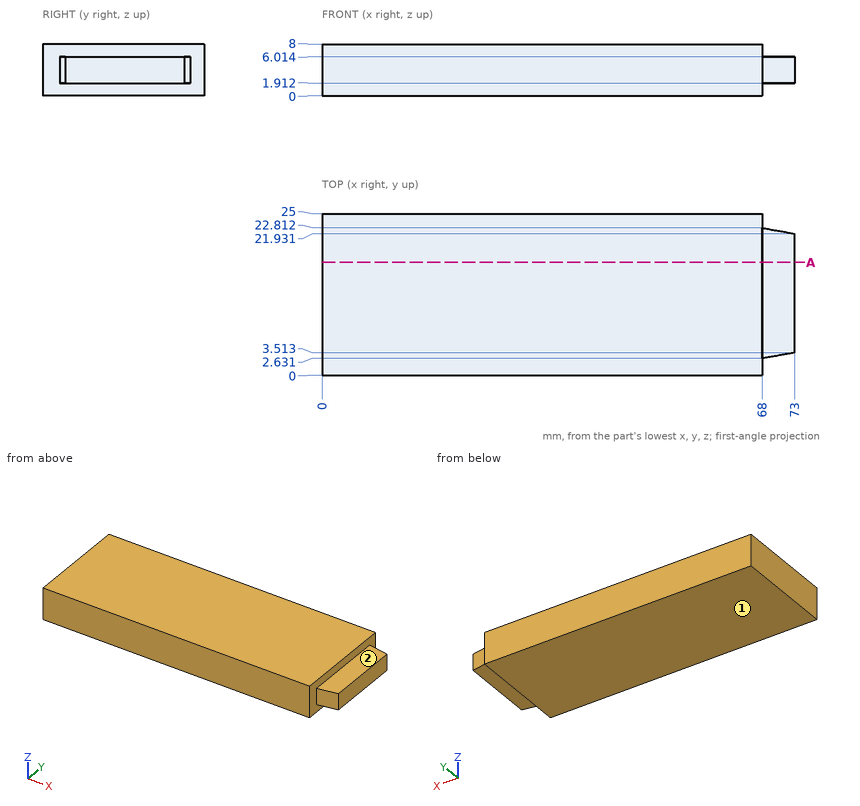
Source: three-view drawing plus pictorial views. Frame: mm from the lowest corner of the part. A direction names the side the tool comes from. Give positions to 0.01 mm unless a question says otherwise; leave off trailing zeros. Write each loop counter-clockwise with the first axis right and the second up, starting at its lowest first coordinate (ties: lowest second). Pieces come first, ordered by that corner, then holes. Notation, with made-up numbers: (10, 24.25) -> (61, 24.25) arc R23 cw to (61, 41.25) -> close; hole circle Ø10 at (48, 17). An arc over 180 degrees is marked (long way). Write item = value, one per line.
Q1. Reachability of the marked faces 1 and 2 from +Z, -Z, +X, -X, +Y, -Y: full face, straight path, thin tool, end or side. Return the list, or none.
Here are the results:
face_1 = -Z, +X, -X, +Y, -Y
face_2 = +Z, +X, +Y, -Y
Q2. First-contact query: pin 1 (4 mm diameter, centred on x = 71.5, y = 14, fed in from -Z). Flat tip, straight axial feed; report the tip coordinate or a pass-through.
Here are the results:
pin_1 = 1.91
Q3. Line query: line 1 (X direction, y = 23.25, z = 2.75); line 2 (Z direction, x = 69, y = 20.25) (1 decimal). Output: solid intervals per line, ascending. Write a range as from..to.
Here are the results:
line_1 = 0..68
line_2 = 1.9..6
Q4. Cut plane A-A on y = 17.5. Return loops of the section in (x, z) (1 decimal).
Here are the results:
outline = (0, 0) -> (68, 0) -> (68, 1.9) -> (73, 1.9) -> (73, 6) -> (68, 6) -> (68, 8) -> (0, 8) -> close
